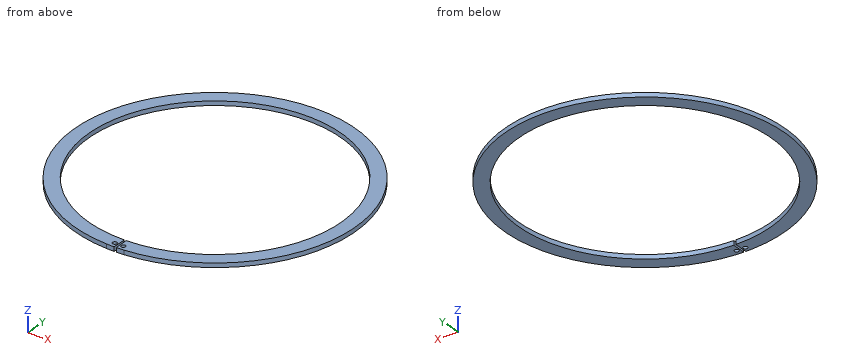
```python
from build123d import *

# Parameters (mm, degrees)
BODYSKE_R   = 2.5
BODY_DEPTH  = 5
UNLUG_DEPTH = 5


with BuildPart() as part:
    # BodySke → Body (new body)
    with BuildSketch(Plane.XY):
        with BuildLine():
            Line((1.125154131, -145.995664416), (1.25, -162.195183344))
            ThreePointArc((1.25, -162.195183344), (5.676371918, -162.100644051), (10.098514589, -161.885329796))
            ThreePointArc((10.098514589, -161.885329796), (10.563651318, -161.684989651), (10.7954035, -161.23467945))
            Line((10.7954035, -161.23467945), (10.957598268, -160.002687876))
            ThreePointArc((10.957598268, -160.002687876), (13.335118636, -155.229150535), (18.145600866, -152.92729855))
            ThreePointArc((18.145600866, -152.92729855), (0, 162), (-18.145600866, -152.92729855))
            ThreePointArc((-18.145600866, -152.92729855), (-13.335118636, -155.229150535), (-10.957598268, -160.002687876))
            Line((-10.957598268, -160.002687876), (-10.7954035, -161.23467945))
            ThreePointArc((-10.7954035, -161.23467945), (-10.563651318, -161.684989651), (-10.098514589, -161.885329796))
            ThreePointArc((-10.098514589, -161.885329796), (-5.676371918, -162.100644051), (-1.25, -162.195183344))
            Line((-1.25, -162.195183344), (-1.125154131, -145.995664416))
            ThreePointArc((-1.125154131, -145.995664416), (0, 146), (1.125154131, -145.995664416))
        make_face()
        with Locations((5, -156.019902577)):
            Circle(BODYSKE_R, mode=Mode.SUBTRACT)
        with Locations((-5, -156.019902577)):
            Circle(BODYSKE_R, mode=Mode.SUBTRACT)
    extrude(amount=-BODY_DEPTH)

    # UnlSke → Unlug (add, through all)
    with BuildSketch(Plane.XY):
        with BuildLine():
            Line((-7.791082109, -162.01277431), (-7.012934574, -145.831473793))
            ThreePointArc((-7.012934574, -145.831473793), (0, 146), (7.012934574, -145.831473793))
            Line((7.012934574, -145.831473793), (7.791082109, -162.01277431))
            ThreePointArc((7.791082109, -162.01277431), (0, 162.2), (-7.791082109, -162.01277431))
        make_face()
    extrude(amount=-UNLUG_DEPTH)


solid = part.part
```
Source: CAD feature listing. Evaluate the final solid. Frame: model axes, mm. Coordinates: 2 decimals unless noted, no trailing zeros. Write each loop counter-clockwise with the first axis right and the second up, starting at its lowest first coordinate (ties: lowest second). Pieces come first, ordered by that corner, then holes. Notation, with made-up numbers: (84.5, -4) - (115.5, -4) arc R12 ccw to (115.5, 3) - close; hole circle Ø7 at (68.5, 30.5). An arc over 180 degrees is marked (long way). Answer as a JSON object with one key per item and string values.
Q1. Section query B-B, the plane x = 93. Output: boundary loops of the cut face in (y, z), plus the area to 3 significant figures.
Ans:
{"outline": "(-132.89, -5) - (-112.55, -5) - (-112.55, 0) - (-132.89, 0) - close; (112.55, -5) - (132.89, -5) - (132.89, 0) - (112.55, 0) - close", "area": "203 mm2"}
Q2. Material intervals for line 1 (X direction, y = 0, z = -1.3); line 2 (Y direction, x = -6.5, z = -2.6); line 3 (Y direction, x = -5, z = -1.35), sorted ascending. Write a range as [from, to].
Ans:
{"line 1": "x = [-162.2, -146], [146, 162.2]", "line 2": "y = [-162.07, -158.02], [-154.02, -145.86], [145.86, 162.07]", "line 3": "y = [-162.12, -158.52], [-153.52, -145.91], [145.91, 162.12]"}
Q3. First-contact query: pin 1 Ø1 at (x, z) = (-63, -4) entering from -Y; pin 2 Ø1.5 at (x, z) = (-59, -4.5) entering from +Y. Flat tips, straight axial feed; report the tip coordinate or a pass-through.
Ans:
{"pin 1": "stops at y = -149.67", "pin 2": "stops at y = 151.38"}
Q4. Section query C-C, the plane z = -3.6. Output: boundary loops of the cut face in (x, y), plus the area to 3 significant figures.
Ans:
{"outline": "(-10.1, -161.89) arc R162.2 ccw to (-1.25, -162.2) - (-1.13, -146) arc R146 cw (long way) to (1.13, -146) - (1.25, -162.2) arc R162.2 ccw to (10.1, -161.89) arc R162.2 ccw (long way) to start; hole circle Ø5 at (-5, -156.02); hole circle Ø5 at (5, -156.02)", "area": "15,600 mm2"}
Q5. Section query A-A, the plane y = 0. Output: boundary loops of the cut face in (x, z), plus the area to 3 significant figures.
Ans:
{"outline": "(-162.2, -5) - (-146, -5) - (-146, 0) - (-162.2, 0) - close; (146, -5) - (162.2, -5) - (162.2, 0) - (146, 0) - close", "area": "162 mm2"}
